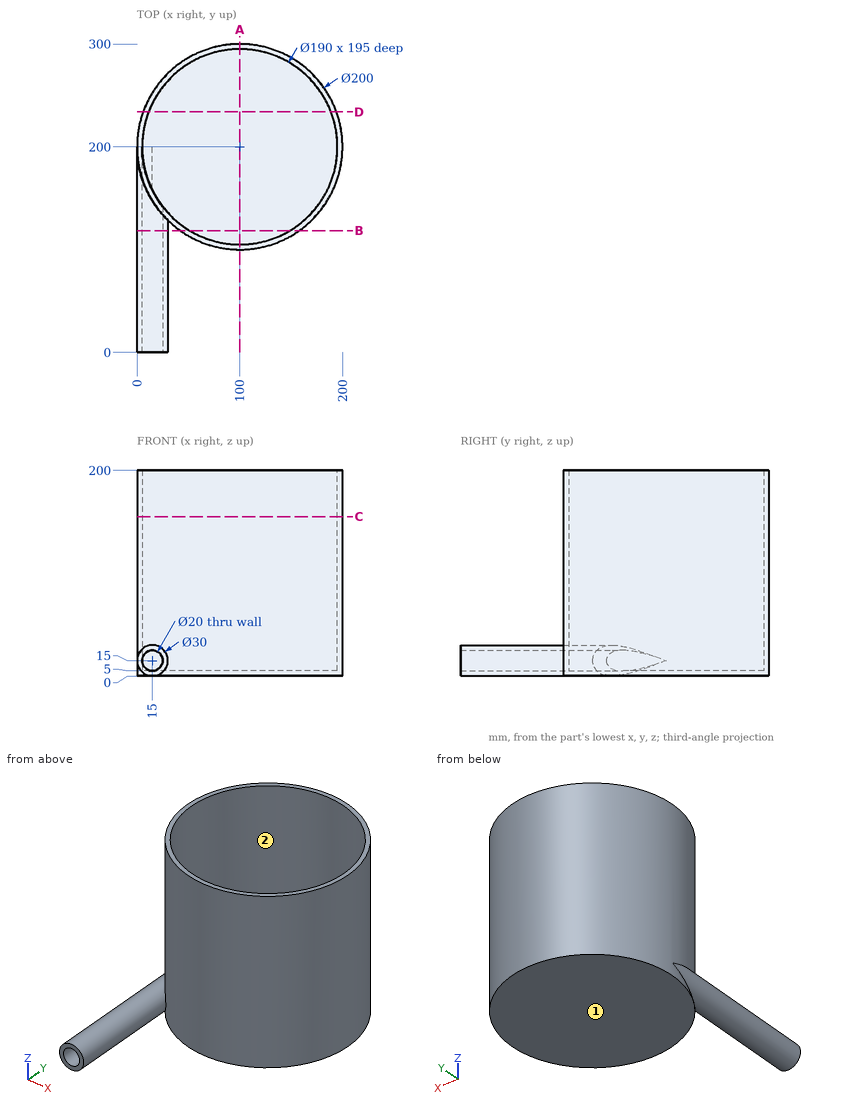
Check sheet for the drawn part. Datum: minimum x, y, z corner. Units: mm. Coordinates: 2 decimals unless noted, no trailing zeros. Loops run counter-clockwise (first coordinate to the right, second up) from the corner with the lowest first, then second, coordinate; pieces in that order, holes last. Notation, with made-up numbers: (16.5, -21) -> (63.5, -21) arc R22 ccw to (63.5, -13) -> close; hole circle Ø7 at (7, 18). An arc over 180 degrees is marked (long way). Answer as a JSON object with one key per item and string values. Group by question number.
Item 1: Scan lines: probe 1 along Z at (x, y) = (15, 110); probe 2 along Y at (x, z) = (100, 128.5); probe 3 along Z at (x, y) = (103, 210.5). Record each from-to range of solid material in increasing order.
Item 2: Sectioned sample at A-A on x = 100. Record the boundary of the cut face in (y, z).
Item 3: Sectioned sample at B-B on y = 118.5. Record the boundary of the cut face in (x, z), plus the area to 3 significant figures.
Item 4: Sectioned sample at D-D on y = 234. Record the boundary of the cut face in (x, z).
Item 5: Sectioned sample at C-C on z = 155. Record the boundary of the cut face in (x, y).
Item 6: Mould release check, pull along X, two halves, no side actions. Record for the marked faces 1 and 2: +X half, -X half, draft (parallel to the pull), parting line (faces both ways), or undercut.
Item 7: Depth check by flat-ended pin: pin 1 (3 mm diameter, centred on y = 185.5, z = 129, fed in from -X); pin 2 (5 mm diameter, centred on x = 90, z = 126.5, fed in from -Y); pin 3 (5 mm diameter, centred on x = 48.5, z = 29, fed in from +Y). Enter the tip coordinate at first touch or a pass-through.
Evaluation:
{
 "1": {"probe 1": "z = 0 to 5, 25 to 30", "probe 2": "y = 100 to 105, 295 to 300", "probe 3": "z = 0 to 5"},
 "2": {"outline": "(100, 0) -> (300, 0) -> (300, 200) -> (295, 200) -> (295, 5) -> (105, 5) -> (105, 200) -> (100, 200) -> close"},
 "3": {"outline": "circle Ø30 at (15, 15); (42.05, 0) -> (157.95, 0) -> (157.95, 200) -> (148.81, 200) -> (148.81, 5) -> (51.19, 5) -> (51.19, 200) -> (42.05, 200) -> close; hole circle Ø20 at (15, 15)", "area": "4,530 mm²"},
 "4": {"outline": "(5.96, 0) -> (194.04, 0) -> (194.04, 200) -> (188.71, 200) -> (188.71, 5) -> (11.29, 5) -> (11.29, 200) -> (5.96, 200) -> close"},
 "5": {"outline": "circle Ø200 at (100, 200); hole circle Ø190 at (100, 200)"},
 "6": {"face 1": "draft", "face 2": "undercut"},
 "7": {"pin 1": "stops at x = 0.85", "pin 2": "stops at y = 100.28", "pin 3": "stops at y = 287.17"}
}
